```python
from build123d import *

# Parameters (mm, degrees)
SKETCH_1_W          = 272.533053494
SKETCH_1_H          = 136.587531522
EXTRUDE_1_DEPTH     = 4
SKETCH_2_W          = 272.533053494
SKETCH_2_H          = 136.587531522
CUT_EXTRUDE_1_DEPTH = 4
CUT_EXTRUDE_2_DEPTH = 4
CUT_EXTRUDE_3_DEPTH = 4
SKETCH_5_W          = 34
SKETCH_5_H          = 36
EXTRUDE_2_DEPTH     = 4
SKETCH_6_W          = 13.2
SKETCH_6_H          = 4
EXTRUDE_3_DEPTH     = 5.6
SKETCH_7_W          = 17.2
SKETCH_7_H          = 30.1
EXTRUDE_4_DEPTH     = 4
SKETCH_8_W          = 5
SKETCH_8_H          = 27.5
CUT_EXTRUDE_4_DEPTH = 4
SKETCH_9_W          = 27.5
SKETCH_9_H          = 2.5
CUT_EXTRUDE_5_DEPTH = 4
SKETCH_10_R         = 1.6
CUT_EXTRUDE_6_DEPTH = 10
EXTRUDE_5_DEPTH     = 190
SKETCH_13_W         = 20
SKETCH_13_H         = 10
CUT_EXTRUDE_7_DEPTH = 300
SKETCH_16_W         = 123.462838452
SKETCH_16_H         = 44.826507499
CUT_EXTRUDE_8_DEPTH = 21
FILLET_2_R          = 5


with BuildPart() as part:
    # 草图1 → 凸台-拉伸1 (new body)
    with BuildSketch(Plane(origin=(0, 0, 0), x_dir=(1, 0, 0), z_dir=(0, 1, 0))):
        Rectangle(SKETCH_1_W, SKETCH_1_H)
    extrude(amount=EXTRUDE_1_DEPTH)

    # 草图2 → 切除-拉伸1 (cut)
    with BuildSketch(Plane(origin=(0, 4, 0), x_dir=(1, 0, 0), z_dir=(0, 1, 0))):
        Rectangle(SKETCH_2_W, SKETCH_2_H)
        with BuildLine():
            Line((-87, 58), (87, 58))
            ThreePointArc((87, 58), (92.656854249, 55.656854249), (95, 50))
            Line((95, 50), (95, -50))
            ThreePointArc((95, -50), (92.656854249, -55.656854249), (87, -58))
            Line((87, -58), (-87, -58))
            ThreePointArc((-87, -58), (-92.656854249, -55.656854249), (-95, -50))
            Line((-95, -50), (-95, 50))
            ThreePointArc((-95, 50), (-92.656854249, 55.656854249), (-87, 58))
        make_face(mode=Mode.SUBTRACT)
    extrude(amount=-CUT_EXTRUDE_1_DEPTH, mode=Mode.SUBTRACT)

    # 草图3 → 切除-拉伸2 (cut)
    with BuildSketch(Plane.XZ):
        Polygon((-95, -22), (-81.8, -22), (-81.8, -19), (-51.8, -19), (-51.8, -46.5), (-81.8, -46.5), (-81.8, -43.5), (-95, -43.5), align=None)
    extrude(amount=-CUT_EXTRUDE_2_DEPTH, mode=Mode.SUBTRACT)

    # 草图4 → 切除-拉伸3 (cut)
    with BuildSketch(Plane.XZ):
        Polygon((-51.5, -18.7), (-51.5, -46.8), (-82.1, -46.8), (-82.1, -43.8), (-95, -43.8), (-95, -21.7), (-82.1, -21.7), (-82.1, -18.7), align=None)
    extrude(amount=-CUT_EXTRUDE_3_DEPTH, mode=Mode.SUBTRACT)

    # 草图5 → 凸台-拉伸2 (add)
    with BuildSketch(Plane.XZ):
        with Locations((-64.8, -32.75)):
            Rectangle(SKETCH_5_W, SKETCH_5_H)
    extrude(amount=EXTRUDE_2_DEPTH)

    # 草图6 → 凸台-拉伸3 (add)
    with BuildSketch(Plane.XZ):
        with Locations((-88.4, -19.7)):
            Rectangle(SKETCH_6_W, SKETCH_6_H)
        with Locations((-88.4, -45.8)):
            Rectangle(SKETCH_6_W, SKETCH_6_H)
    extrude(amount=EXTRUDE_3_DEPTH)

    # 草图7 → 凸台-拉伸4 (add)
    with BuildSketch(Plane.XZ.offset(5.6)):
        with Locations((-86.4, -32.75)):
            Rectangle(SKETCH_7_W, SKETCH_7_H)
    extrude(amount=EXTRUDE_4_DEPTH)

    # 草图8 → 切除-拉伸4 (cut)
    with BuildSketch(Plane(origin=(0, 4, 0), x_dir=(1, 0, 0), z_dir=(0, 1, 0))):
        with Locations((-43.3, 32.75)):
            Rectangle(SKETCH_8_W, SKETCH_8_H)
    extrude(amount=-CUT_EXTRUDE_4_DEPTH, mode=Mode.SUBTRACT)

    # 草图9 → 切除-拉伸5 (cut)
    with BuildSketch(Plane(origin=(-45.8, 0, 0), x_dir=(0, 0, -1), z_dir=(1, 0, 0))):
        with Locations((32.75, 2.75)):
            Rectangle(SKETCH_9_W, SKETCH_9_H)
    extrude(amount=-CUT_EXTRUDE_5_DEPTH, mode=Mode.SUBTRACT)

    # 草图10 → 切除-拉伸6 (cut)
    with BuildSketch(Plane(origin=(0, 4, 0), x_dir=(1, 0, 0), z_dir=(0, 1, 0))):
        with Locations(Location((87.4, 50.9, 0), (0, 0, 270))):
            Circle(SKETCH_10_R)
        with Locations(Location((-87.4, 50.9, 0), (0, 0, 270))):
            Circle(SKETCH_10_R)
        with Locations(Location((-87.4, -50.9, 0), (0, 0, 270))):
            Circle(SKETCH_10_R)
        with Locations(Location((87.4, -50.9, 0), (0, 0, 270))):
            Circle(SKETCH_10_R)
    extrude(amount=-CUT_EXTRUDE_6_DEPTH, mode=Mode.SUBTRACT)

    # 草图11 → 凸台-拉伸5 (add)
    with BuildSketch(Plane(origin=(95, 0, 0), x_dir=(0, 0, -1), z_dir=(1, 0, 0))):
        Polygon((0.198533436, 0.024346469), (-29.801466564, 0), (-17.394200934, -14.762056921), align=None)
    extrude(amount=-EXTRUDE_5_DEPTH)

    # 草图13 → 切除-拉伸7 (cut)
    with BuildSketch(Plane(origin=(0, -14.678538072, 17.464397151), x_dir=(1, 0, 0), z_dir=(0, -0.6434090803775565, 0.7655225374133063))):
        with Locations((79.5, 8.890899555)):
            Rectangle(SKETCH_13_W, SKETCH_13_H)
        with Locations((-79.5, 8.890899555)):
            Rectangle(SKETCH_13_W, SKETCH_13_H)
    extrude(amount=-CUT_EXTRUDE_7_DEPTH, mode=Mode.SUBTRACT)

    # 草图16 → 切除-拉伸8 (cut)
    with BuildSketch(Plane.XZ):
        with Locations((0, 10.193598456)):
            Rectangle(SKETCH_16_W, SKETCH_16_H)
    extrude(amount=CUT_EXTRUDE_8_DEPTH, mode=Mode.SUBTRACT)

    # 圆角2
    fillet_2_edges = [part.edges().sort_by_distance(p)[0] for p in [
        (-78.365709613, 0, 29.801466564),
        (-78.365709613, 0, -0.169566218),
        (78.365709613, 0, -0.169566218),
        (78.365709613, 0, 29.801466564),
        (61.731419226, 0, 14.815950173),
        (-61.731419226, 0, 14.815950173),
    ]]
    fillet(fillet_2_edges, radius=FILLET_2_R)


solid = part.part
```
Check sheet for the modelled part. Datum: model origin and axes. Units: mm. A direction names the side the tool comes from. Round coordinates to 2 decimals unless told otherwise and drop trailing zeros. Write each loop counter-clockwise with the first axis right and the second up, starting at its lowest first coordinate (ties: lowest second). Pieces come first, ordered by that corner, then holes. Notation, with made-up numbers: (65, 71.5) -> (116, 71.5) arc R31 ccw to (116, 110.5) -> close; hole circle Ø9 at (37, 69). An arc over 180 degrees is marked (long way). One line per question, with ' | ' between items. Start each with the question number.
1. Set-up check for faces 4 (the face through (60.2, -1.4, 15.3)), 5 (the face through (-87, -5, -17.7)), 6 (the face through (-87, -5, -47.8)), 7 (the face through (-65, -2, -14.75)), 8 (the face through (-67, 2, -46.8)): record each of +Z, -Z, +X, -X, +Y, -Y from which the full face is reachable in a straight line by a thin tool's end or side.
2. Release check for a two-part mould opening along Z. For faces 1 (the face through (-92.594, 2.028, 55.719)), 2 (the face through (-67, 2, -18.7)), 3 (the face through (61.731, -9, 16)) record: +Z half, -Z half, draft (parallel to the pull), parting line (faces both ways), or undercut.
3. Sectioned sample at C-C, the plane z = -8.5. Record the cut outline in (x, y).
4. Sectioned sample at A-A, the plane z = -41. Record the cut outline in (x, y).
5. Depth check by flat-ended pin: pin 1 (8 mm diameter, centred on x = -75.5, y = -4.5, fed in from +Z); pin 2 (1.5 mm diameter, centred on y = -2.5, z = -16.5, fed in from -X); pin 3 (1.5 mm diameter, centred on x = -42, z = 37, fed in from -Y); pin 4 (3.5 mm diameter, centred on x = 87.4, z = 50.9, fed in from +Y). Enter the tip coordinate at first touch or a pass-through.
6. Sectioned sample at B-B, the plane z = 22. Record the cut outline in (x, y) (3 decimals), then the cut area to 3 significant figures.
7. Scan lines: line 1 along X through (y, z) = (2.95, 50.9); line 2 along X through (y, z) = (0.75, 11); line 3 along Z through (x, y) = (87.4, 2.3). Record each from-to range of solid material in increasing order. Write a range as from..to.
Taken from the geometry:
1) face 4: +Z, -Z, -Y | face 5: -X, -Y | face 6: -Z, -X, -Y | face 7: +X, -X, -Y | face 8: +Y
2) face 1: +Z half | face 2: undercut | face 3: draft
3) outline: (-95, 0) -> (95, 0) -> (95, 4) -> (-95, 4) -> close
4) outline: (-95, -9.6) -> (-77.8, -9.6) -> (-77.8, -5.6) -> (-95, -5.6) -> close; (-81.8, -4) -> (-47.8, -4) -> (-47.8, 0) -> (-45.8, 0) -> (-45.8, 1.5) -> (-49.8, 1.5) -> (-49.8, 4) -> (-51.5, 4) -> (-51.5, 0) -> (-81.8, 0) -> close; (-40.8, 0) -> (95, 0) -> (95, 4) -> (-40.8, 4) -> close
5) pin 1: stops at z = 29.95 | pin 2: stops at x = -81.8 | pin 3: stops at y = 0 | pin 4: stops at y = 4
6) outline: (-95, -9.282) -> (-89.5, -9.282) -> (-89.5, -0.345) -> (-69.5, -0.345) -> (-69.5, -9.282) -> (-61.731, -9.282) -> (-61.731, -5) arc R5 cw to (-56.731, 0) -> (56.731, 0) arc R5 cw to (61.731, -5) -> (61.731, -9.282) -> (69.5, -9.282) -> (69.5, -0.345) -> (89.5, -0.345) -> (89.5, -9.282) -> (95, -9.282) -> (95, 4) -> (-95, 4) -> close | area: 1,030 mm^2
7) line 1: x = -94.95..-89, -85.8..85.8, 89..94.95 | line 2: x = -95..-89.5, -69.5..69.5, 89.5..95 | line 3: z = -57.99..-52.5, -49.3..3.31, 18.85..49.3, 52.5..57.99
